```python
from build123d import *

# Parameters (mm, degrees)
F1_DEPTH = 3.175
F2_R     = 2.4257
F3_DEPTH = 12.7
F4_R     = 1.1938
F5_DEPTH = 2.3876


with BuildPart() as f1:
    # F0 (on Front) → F1 (new body)
    with BuildSketch(Plane.XZ):
        with BuildLine():
            Line((-28.943281, 4.662325), (-28.87206, 4.661781))
            ThreePointArc((-28.87206, 4.661781), (-28.907669, 4.662189), (-28.943281, 4.662325))
        make_face()
        with BuildLine():
            Line((-0.656047, 4.446255), (-28.87206, 4.661781))
            Line((-28.87206, 4.661781), (-28.943281, 4.662325))
            ThreePointArc((-28.943281, 4.662325), (-33.605606, 0), (-28.943281, -4.662325))
            Line((-28.943281, -4.662325), (-0.655231, -4.446375))
            ThreePointArc((-0.655231, -4.446375), (4.494394, 0.000412), (-0.656047, 4.446255))
        make_face()
    extrude(amount=F1_DEPTH)

    # F2 (on face) → F3 (join)
    with BuildSketch(Plane.XZ.offset(3.175)):
        Circle(F2_R)
    extrude(amount=F3_DEPTH)

    # F4 (on face) → F5 (join)
    with BuildSketch(Plane(origin=(0, 0, 0), x_dir=(-1, 0, 0), z_dir=(0, 1, 0))):
        with Locations((28.943281, 0)):
            Circle(F4_R)
        with Locations((12.433281, 0)):
            Circle(F4_R)
    extrude(amount=F5_DEPTH)


solid = f1.part
```
Verification items for the finished model (mm, model axes). A direction names the side the tool comes from. Coordinates: 2 decimals unless noted, no trailing zeros. Loops run counter-clockwise (first coordinate to the right, second up) from the corner with the lowest first, then second, coordinate; pieces in that order, holes last. Notation, with made-up numbers: (14.5, -14) - (42.5, -14) arc R17 cw to (42.5, 13) - close; hole circle Ø6 at (75.25, 30.25). An arc over 180 degrees is marked (long way). Return JSON: item names as keys, results as strings.
1. Thickness scan on L1, parallel to Y at x = -8, z = -1.5 (3 decimals); L2, parallel to X at y = -4.5, z = -2; L3, parallel to X at y = -3.25, z = 1. Record the ranges inside material, lowest first.
Established:
{"L1": "y = -3.175 to 0", "L2": "x = -1.37 to 1.37", "L3": "x = -2.21 to 2.21"}
2. Section check D-D, the plane x = -7.5. Record the boundary of the cut face in (y, z) (3 decimals), then the cut area to 3 significant figures.
Established:
{"outline": "(-3.175, -4.499) - (0, -4.499) - (0, 4.499) - (-3.175, 4.499) - close", "area": "28.6 mm2"}
3. Section check B-B, the plane y = -1. Record the boundary of the cut face in (x, z), then the cut area to 3 significant figures.
Established:
{"outline": "(-28.94, -4.66) - (-0.66, -4.45) arc R4.49 ccw (long way) to (-0.66, 4.45) - (-28.87, 4.66) arc R4.66 ccw to (-28.94, 4.66) arc R4.66 ccw to start", "area": "329 mm2"}
4. Go/stop test with flat-tipped pins: pin 1 (3 mm diameter, centred on x = -15, z = -3.5, fed in from -Y) (3 decimals); pin 2 (1.5 mm diameter, centred on x = -13, y = -1, fed in from +Z); pin 3 (1 mm diameter, centred on y = -4, z = -1, fed in from -X). Record where each tip stops, or that it passes through.
Established:
{"pin 1": "stops at y = -3.175", "pin 2": "stops at z = 4.55", "pin 3": "stops at x = -2.37"}
5. Section check A-A, the plane z = 0. Record the boundary of the cut face in (x, y) (3 decimals), then the cut area to 3 significant figures.
Established:
{"outline": "(-33.606, -3.175) - (-2.426, -3.175) - (-2.426, -15.875) - (2.426, -15.875) - (2.426, -3.175) - (4.494, -3.175) - (4.494, 0) - (-11.239, 0) - (-11.239, 2.388) - (-13.627, 2.388) - (-13.627, 0) - (-27.749, 0) - (-27.749, 2.388) - (-30.137, 2.388) - (-30.137, 0) - (-33.606, 0) - close", "area": "194 mm2"}
6. Section check C-C, the plane x = 0. Record the boundary of the cut face in (y, z) (3 decimals), then the cut area to 3 significant figures.
Established:
{"outline": "(-15.875, -2.426) - (-3.175, -2.426) - (-3.175, -4.494) - (0, -4.494) - (0, 4.494) - (-3.175, 4.494) - (-3.175, 2.426) - (-15.875, 2.426) - close", "area": "90.2 mm2"}
7. Tool access check on faces 1 (the cylindrical face through (-30.08, 1.18, 0.36)), 2 (the flat face through (0, -15.875, 0)), 3 (the cylindrical face through (2.314, -9.436, 0.729)). Record the directions out of +Z, -Z, +X, -X, +Y, -Y that give a thin tool (end or side, any length) a straight path to the whole face; none if there is none.
Established:
{"face 1": "+Y", "face 2": "+Z, -Z, +X, -X, -Y", "face 3": "-Y"}
